Model file for the job. Use its own axes, mm. Face numbers are marked on the shaded views. A direction names the side the tool comes from. Give positions to 0.01 mm unless a question says otherwise; leave off trailing zeros. Order: outer loops, then holes, each group sorted by start corner. A loop starts at its lowest first (then second) coordinate and runs counter-clockwise, first axis right, second up. Notation, with made-up numbers: (-36, -19.75) -> (-17, -19.75) arc R30 ccw to (-17, 13.25) -> close; hole circle Ø5 at (-34, 23). An arc over 180 degrees is marked (long way). Use CSV: the item, a comma, the result in double quotes. Start each with the question number.
1. Cut at C-C on y = 32.5. List the corners of the cut face in (x, z).
2. Cut at D-D on x = 48. Give the number of separate pieces and of enclosed holes in the cut face, then the cut area to 3 significant figures.
3. Pull direction Y, two halves, no side cores. Call the marked faces 1, 2 and 3: released by +Y, released by -Y, zero draft, split by the parting line, or undercut.
4. 3-axis set-ups, long thin cutter, end or side, ignore diameter. For the marked faces 4, 5, 6, 7 and 8: which of +Z, -Z, +X, -X, +Y, -Y reach the whole face in a straight line?
5. Cut at A-A on x = 32. List the corners of the cut face in (y, z), then the cut area to 3 significant figures.
6. Drop flat-ended pins along their axis: pin 1 (3 mm diameter, centred on x = 56, y = 40, fed in from +Z); pin 2 (5.5 mm diameter, centred on x = 79.5, z = 27, fed in from +Y); pin 3 (1.5 mm diameter, centred on x = 51.5, y = -2.5, fed in from +Z); pin 4 (10 mm diameter, centred on x = 51.5, z = 18.5, fed in from +Y). Give the stop position or say it passes through.
7. Wall check: line 1 (X direction, y = 48, z = 22.5); line 2 (Y direction, x = 77.5, z = 2.5); line 3 (Z direction, x = 46.5, y = 34.5). Give the ranges that are in metal, low to high. Write a range as from..to.
Solid Edge part; units mm, degrees
sketch "Sketch1" plane through (0, 0, 0) normal (0, 0, 1) x (1, 0, 0)
  line L0 (18.6142, 0) -> (82.6142, 0)
  line L1 (82.6142, 0) -> (82.6142, 64)
  line L2 (82.6142, 64) -> (18.6142, 64)
  line L3 (18.6142, 64) -> (18.6142, 0)
extrude "Protrusion1" add sketch "Sketch1" along normal blind 34
sketch "Sketch2" plane through (50.6142, 32, 34) normal (0, 0, 1) x (1, 0, 0)
  line L0 (-27, 27) -> (27, 27)
  line L1 (27, 27) -> (27, -27)
  line L2 (27, -27) -> (-27, -27)
  line L3 (-27, -27) -> (-27, 27)
  dimension "D1" = 27
  dimension "D2" = 27
  dimension "D3" = 27
extrude "ExtrudedCutout_1" cut sketch "Sketch2" against normal blind 31
sketch "Sketch3" plane through (50.6142, 32, 34) normal (0, 0, 1) x (0, 1, 0)
  line L0 (-17, 32) -> (-17, 27)
  line L1 (-17, 27) -> (17, 27)
  line L2 (17, 27) -> (17, 32)
  line L3 (17, 32) -> (-17, 32)
  line L4 (-17, -27) -> (17, -27)
  line L5 (17, -27) -> (17, -32)
  line L6 (17, -32) -> (-17, -32)
  line L7 (-17, -32) -> (-17, -27)
extrude "ExtrudedCutout_3" cut sketch "Sketch3" against normal blind 10
sketch "Sketch4" plane through (50.6142, 0, 17) normal (0, -1, 0) x (1, 0, 0)
  circle A0 centre (0, 0) radius 14
extrude "Protrusion2" add sketch "Sketch4" along normal blind 20
sketch "Sketch5" plane through (50.6142, 64, 17) normal (0, 1, 0) x (-1, 0, 0)
  circle A0 centre (0, 0) radius 14
extrude "ExtrudedProtrusion_3" add sketch "Sketch5" along normal blind 20
fillet "Round_1" radius 6 4 edges at (23.6142, 5, 18.5) (23.6142, 59, 18.5) (77.6142, 59, 18.5) (77.6142, 5, 18.5)
hole "Hole_4" at (50.6142, 84, 17) direction (0, -1, 0) diameter 22.835 end up to next thread major 25 thread length 6
hole "Hole_5" at (50.6142, -20, 17) direction (0, 1, 0) diameter 22.835 end up to next thread major 25 thread length 6
fillet "Round_2" radius 3 2 edges at (64.6142, 64, 17) (36.6142, 0, 17)
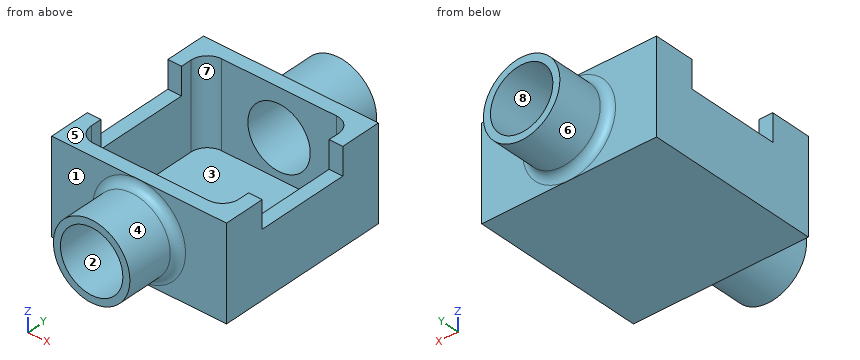
Verdict:
1,outline,"(18.61, 0) -> (82.61, 0) -> (82.61, 24) -> (77.61, 24) -> (77.61, 3) -> (23.61, 3) -> (23.61, 24) -> (18.61, 24) -> close"
2,separate pieces,"3"
2,enclosed holes,"0"
2,area,"499 mm^2"
3,face 1,"released by -Y"
3,face 2,"zero draft"
3,face 3,"undercut"
4,face 4,"-Y"
4,face 5,"+Z, +X, -X, +Y, -Y"
4,face 6,"+Y"
4,face 7,"+Z"
4,face 8,"+Y, -Y"
5,outline,"(0, 0) -> (64, 0) -> (64, 34) -> (59, 34) -> (59, 3) -> (5, 3) -> (5, 34) -> (0, 34) -> close"
5,area,"502 mm^2"
6,pin 1,"z = 3"
6,pin 2,"y = 64"
6,pin 3,"z = 31.25"
6,pin 4,"through"
7,line 1,"18.61..23.61, 77.61..82.61"
7,line 2,"0..64"
7,line 3,"0..3"
